```python
from build123d import *

# Parameters (mm, degrees)
SKETCH2_R               = 5
BOSS_EXTRUDE2_DEPTH     = 50
FILLET1_R               = 10
CUT_EXTRUDE1_DEPTH      = 195.993878356
CUT_EXTRUDE1_DEPTH_BACK = 195.993878356
SKETCH3_W               = 20
SKETCH3_H               = 86.120343404
SKETCH4_R               = 5
CUT_EXTRUDE2_DEPTH      = 156.50648845


with BuildPart() as part:
    # Sketch2 → Boss-Extrude2 (new body)
    with BuildSketch(Plane.XY):
        Polygon((0, 120), (-45, 120), (-87.945471533, 89.9292571), (-60, 30), (-60, 0), (0, 0), (60, 0), (60, 30), (87.945471533, 89.9292571), (45, 120), align=None)
        with Locations((-50.289922216, 105.614178936)):
            Circle(SKETCH2_R, mode=Mode.SUBTRACT)
        with Locations((-76.912363656, 86.972944754)):
            Circle(SKETCH2_R, mode=Mode.SUBTRACT)
        with Locations(Location((76.912363656, 86.972944754, 0), (0, 0, 180))):
            Circle(SKETCH2_R, mode=Mode.SUBTRACT)
        with Locations(Location((50.289922216, 105.614178936, 0), (0, 0, 180))):
            Circle(SKETCH2_R, mode=Mode.SUBTRACT)
        Polygon((0, 102.5), (-39.482271195, 102.5), (-65.879255778, 84.016632409), (-42.5, 33.879656596), (42.5, 33.879656596), (65.879255778, 84.016632409), (39.482271195, 102.5), align=None, mode=Mode.SUBTRACT)
    extrude(amount=BOSS_EXTRUDE2_DEPTH)

    # Fillet1
    fillet1_edges = [part.edges().sort_by_distance(p)[0] for p in [
        (-45, 120, 25),
        (45, 120, 25),
        (87.945471533, 89.9292571, 25),
        (60, 30, 25),
        (-60, 30, 25),
        (-87.945471533, 89.9292571, 25),
        (65.879255778, 84.016632409, 25),
        (39.482271195, 102.5, 25),
        (-39.482271195, 102.5, 25),
        (-65.879255778, 84.016632409, 25),
        (-42.5, 33.879656596, 25),
        (42.5, 33.879656596, 25),
    ]]
    fillet(fillet1_edges, radius=FILLET1_R)

    # Sketch3 → Cut-Extrude1 (cut, two sides: drawn at the far end of the back side and taken through both)
    with BuildSketch(Plane.ZY.offset(60).offset(-CUT_EXTRUDE1_DEPTH_BACK)):
        with Locations((25, 76.939828298)):
            Rectangle(SKETCH3_W, SKETCH3_H)
    extrude(amount=CUT_EXTRUDE1_DEPTH + CUT_EXTRUDE1_DEPTH_BACK, mode=Mode.SUBTRACT)

    # Sketch4 → Cut-Extrude2 (cut, through all)
    with BuildSketch(Plane.XZ):
        with Locations(Location((0, 25, 0), (0, 0, 270))):
            Circle(SKETCH4_R)
    extrude(amount=-CUT_EXTRUDE2_DEPTH, mode=Mode.SUBTRACT)


solid = part.part
```
The listing builds one solid part. Answer for the finished solid, in the listing's coordinates (mm). A direction names the side the tool comes from. Give positions to 0.01 mm unless a question says otherwise; leave off trailing zeros. Order: outer loops, then holes, each group sorted by start corner. A loop starts at its lowest first (then second) coordinate and runs counter-clockwise, first axis right, second up. Notation, with made-up numbers: (-36.5, 66) -> (8.5, 66) arc R22 cw to (8.5, 79) -> close; hole circle Ø7 at (89.25, 48.25). An arc over 180 degrees is marked (long way). Answer as a JSON object with one key per item and string values. Group by question number.
Item 1: The part is cut by section A-A on x = -31. Write down the section's boundary in (y, z), and give its area (3 significant figures).
Item 2: Determine the mould class of faces 1 (the flat face through (60, 14, 25)), 2 (the flat face through (-72.832, 57.519, 35.761)), 3 (the flat face through (-1, 102.5, 42)) for opening direction X: pulls with the +X half, pulls with the -X half, needs draft (parallel to the pull), parting line crosses it, or undercut.
Item 3: The part is cut by section C-C on y = 10. Write down the section's boundary in (x, z), and give its area (3 significant figures).
Item 4: The part is cut by section D-D on x = 0. Write down the section's boundary in (y, z).
Item 5: The part is cut by section B-B on z = 25. Write down the section's boundary in (x, y), and give its area (3 significant figures).
Item 6: Flat-ended cylindrical pins translate along their axes: pin 1 (3 mm diameter, centred on y = 25, z = 27.5, fed in from -X); pin 2 (9 mm diameter, centred on x = 76.91, y = 86.97, fed in from -Z); pin 3 (2 mm diameter, centred on x = -31, z = 12, fed in from -Y); pin 4 (3 mm diameter, centred on y = 75, z = 12.5, fed in from +X). Find the tip coordinate at first contact, or state that the pin passes through.
Item 7: A tool of negligible diameter and unlimited length cuts with its end or side. For faces 4 (the cylindrical face through (-39.3, 102.05, 42.6)), 5 (the cylindrical face through (85.02, 89.04, 42.6)), 6 (the flat face through (0, 105, 15)), from which of +Z, -Z, +X, -X, +Y, -Y can it reach the whole face along a straight path? Write none if from no direction.
Item 8: Consider L1, parallel to X at y = 109, z = 5.5; L2, parallel to Z at x = -10.5, y = 107.5; L3, parallel to Y at x = -16.5, z = 38.5. Determine where each line is inside the solid, lowest interval first. Write a range as from..to.
Result set:
{
 "1": {"outline": "(0, 0) -> (33.88, 0) -> (33.88, 50) -> (0, 50) -> close; (102.5, 0) -> (120, 0) -> (120, 15) -> (102.5, 15) -> close; (102.5, 35) -> (120, 35) -> (120, 50) -> (102.5, 50) -> close", "area": "2,220 mm²"},
 "2": {"face 1": "pulls with the +X half", "face 2": "pulls with the -X half", "face 3": "undercut"},
 "3": {"outline": "(-60, 0) -> (60, 0) -> (60, 50) -> (-60, 50) -> close; hole circle Ø10 at (0, 25)", "area": "5,920 mm²"},
 "4": {"outline": "(0, 0) -> (33.88, 0) -> (33.88, 20) -> (0, 20) -> close; (0, 30) -> (33.88, 30) -> (33.88, 50) -> (0, 50) -> close; (102.5, 0) -> (120, 0) -> (120, 15) -> (102.5, 15) -> close; (102.5, 35) -> (120, 35) -> (120, 50) -> (102.5, 50) -> close"},
 "5": {"outline": "(-61.81, 33.88) -> (-60.94, 32.01) arc R10 cw to (-60, 27.78) -> (-60, 0) -> (-5, 0) -> (-5, 33.88) -> close; (5, 0) -> (60, 0) -> (60, 27.78) arc R10 cw to (60.94, 32.01) -> (61.81, 33.88) -> (5, 33.88) -> close", "area": "3,730 mm²"},
 "6": {"pin 1": "x = -60", "pin 2": "through", "pin 3": "y = 0", "pin 4": "x = 81.68"},
 "7": {"face 4": "+Z, -Z", "face 5": "+Z, -Z, +X", "face 6": "+X, -X, +Y"},
 "8": {"L1": "-60.71..-53.97, -46.61..46.61, 53.97..60.71", "L2": "0..15, 35..50", "L3": "0..33.88, 102.5..120"}
}
